Build history of the part. All positions in model axes, mm. Round coordinates to 2 decimals unless told otherwise and drop trailing zeros. Answer as a JSON object with one key per item and string values. Group by question number.
Item 1: Slice it at A-A, the plane z = 1.05. Give the number of separate pieces and of enclosed holes in the cut face, then the cut area to 3 significant figures.
Item 2: Probe line 1 (Y direction, x = 39.1, z = 0.65); line 2 (Y direction, x = -42.9, z = 1.3); line 3 (X direction, y = 20, z = 0.4). List the from-to ranges inside material, lowest first. Write a range as from..to.
Item 3: Two-plate mould, pull along Y, no slides. Class faces 1 (the cylindrical face through (4.316, -19.453, 0.862)), 2 (the flat face through (-3, 1, 1.7)): +Y half, -Y half, draft (parallel to the pull), parting line (faces both ways), or undercut.
Item 4: Flat gauge pins, fed straight in: pin 1 (3.5 mm diameter, centred on x = 0, y = 19.8, fed in from -Z); pin 2 (1.6 mm diameter, centred on x = -224.2, y = 26.5, fed in from -Z); pin 3 (0.5 mm diameter, centred on y = -46.5, z = 0.5, fed in from -X). Where does each tip first touch, or does it go through?
from build123d import *

# Parameters (mm, degrees)
SKETCH3_W           = 458
SKETCH3_H           = 118
BOSS_EXTRUDE2_DEPTH = 1.7
SKETCH4_R           = 1.35
CUT_EXTRUDE1_DEPTH  = 237.484439234
CUT_EXTRUDE2_DEPTH  = 237.484439234
SKETCH6_R           = 9
CUT_EXTRUDE3_DEPTH  = 237.484439234
SKETCH8_W           = 11
SKETCH8_H           = 7
CUT_EXTRUDE4_DEPTH  = 237.484439234


with BuildPart() as part:
    # Sketch3 → Boss-Extrude2 (new body)
    with BuildSketch(Plane.XY):
        Rectangle(SKETCH3_W, SKETCH3_H)
    extrude(amount=BOSS_EXTRUDE2_DEPTH)

    # Sketch4 → Cut-Extrude1 (cut, through all)
    with BuildSketch(Plane.XY.offset(1.7)):
        with Locations((0, 19.8)):
            Circle(SKETCH4_R)
        with Locations((0, -25.5)):
            Circle(SKETCH4_R)
        with Locations((39.1, -55)):
            Circle(SKETCH4_R)
        with Locations((42.9, -26)):
            Circle(SKETCH4_R)
        with Locations((224.2, -55)):
            Circle(SKETCH4_R)
        with Locations(Location((-224.2, -55, 0), (0, 0, 180))):
            Circle(SKETCH4_R)
        with Locations(Location((-42.9, -26, 0), (0, 0, 180))):
            Circle(SKETCH4_R)
        with Locations(Location((-39.1, -55, 0), (0, 0, 180))):
            Circle(SKETCH4_R)
        with Locations((224.2, 46.5)):
            Circle(SKETCH4_R)
        with Locations((224.2, 26.5)):
            Circle(SKETCH4_R)
        with Locations((224.2, 6.5)):
            Circle(SKETCH4_R)
        with Locations((224.2, -13.5)):
            Circle(SKETCH4_R)
        with Locations(Location((-224.2, -13.5, 0), (0, 0, 180))):
            Circle(SKETCH4_R)
        with Locations(Location((-224.2, 6.5, 0), (0, 0, 180))):
            Circle(SKETCH4_R)
        with Locations(Location((-224.2, 26.5, 0), (0, 0, 180))):
            Circle(SKETCH4_R)
        with Locations(Location((-224.2, 46.5, 0), (0, 0, 180))):
            Circle(SKETCH4_R)
    extrude(amount=-CUT_EXTRUDE1_DEPTH, mode=Mode.SUBTRACT)

    # Sketch5 → Cut-Extrude2 (cut, through all)
    with BuildSketch(Plane.XY.offset(1.7)):
        with BuildLine():
            Line((-32, -59), (32, -59))
            Line((32, -59), (32, -34))
            ThreePointArc((32, -34), (30.535533906, -30.464466094), (27, -29))
            Line((27, -29), (-27, -29))
            ThreePointArc((-27, -29), (-30.535533906, -30.464466094), (-32, -34))
            Line((-32, -34), (-32, -59))
        make_face()
    extrude(amount=-CUT_EXTRUDE2_DEPTH, mode=Mode.SUBTRACT)

    # Sketch6 → Cut-Extrude3 (cut, through all)
    with BuildSketch(Plane.XY.offset(1.7)):
        with Locations((-12.9, -16.75)):
            Circle(SKETCH6_R)
        with Locations((-12.9, 10.25)):
            Circle(SKETCH6_R)
        with Locations(Location((12.9, -16.75, 0), (0, 0, 180))):
            Circle(SKETCH6_R)
        with Locations(Location((12.9, 10.25, 0), (0, 0, 180))):
            Circle(SKETCH6_R)
    extrude(amount=-CUT_EXTRUDE3_DEPTH, mode=Mode.SUBTRACT)

    # Sketch8 → Cut-Extrude4 (cut, through all)
    with BuildSketch(Plane.XY.offset(1.7)):
        with Locations((-44.26, -47)):
            Rectangle(SKETCH8_W, SKETCH8_H)
        with Locations((-74.63, -47)):
            Rectangle(SKETCH8_W, SKETCH8_H)
        with Locations((-152, -47)):
            Rectangle(SKETCH8_W, SKETCH8_H)
        with Locations((-228, -47)):
            Rectangle(SKETCH8_W, SKETCH8_H)
        with Locations((228, -47)):
            Rectangle(SKETCH8_W, SKETCH8_H)
        with Locations((152, -47)):
            Rectangle(SKETCH8_W, SKETCH8_H)
        with Locations((74.63, -47)):
            Rectangle(SKETCH8_W, SKETCH8_H)
        with Locations((44.26, -47)):
            Rectangle(SKETCH8_W, SKETCH8_H)
    extrude(amount=-CUT_EXTRUDE4_DEPTH, mode=Mode.SUBTRACT)


solid = part.part
Geometry says:
{
 "1": {"separate pieces": "1", "enclosed holes": "26", "area": "50,500 mm^2"},
 "2": {"line 1": "y = -59..-56.35, -53.65..-50.5, -43.5..59", "line 2": "y = -59..-50.5, -43.5..-27.35, -24.65..59", "line 3": "x = -229..-1.34, 1.34..229"},
 "3": {"face 1": "undercut", "face 2": "draft"},
 "4": {"pin 1": "stops at z = 0", "pin 2": "passes through", "pin 3": "stops at x = -222.5"}
}
